Part print with two shaded views. Sizes in mm from the minimum x, y, z corner. A direction names the side the tool comes from. Round coordinates to 2 decimals unless told otherwise and drop trailing zeros. Loops run counter-clockwise (first coordinate to the right, second up) from the corner with the lowest first, then second, coordinate; pieces in that order, holes last. Notation, with made-up numbers: (20.25, 42) - (54.25, 42) arc R31 cw to (54.25, 70) - close; hole circle Ø4 at (57.5, 1.25). An arc over 180 degrees is marked (long way). Use a Markdown table: item, result.
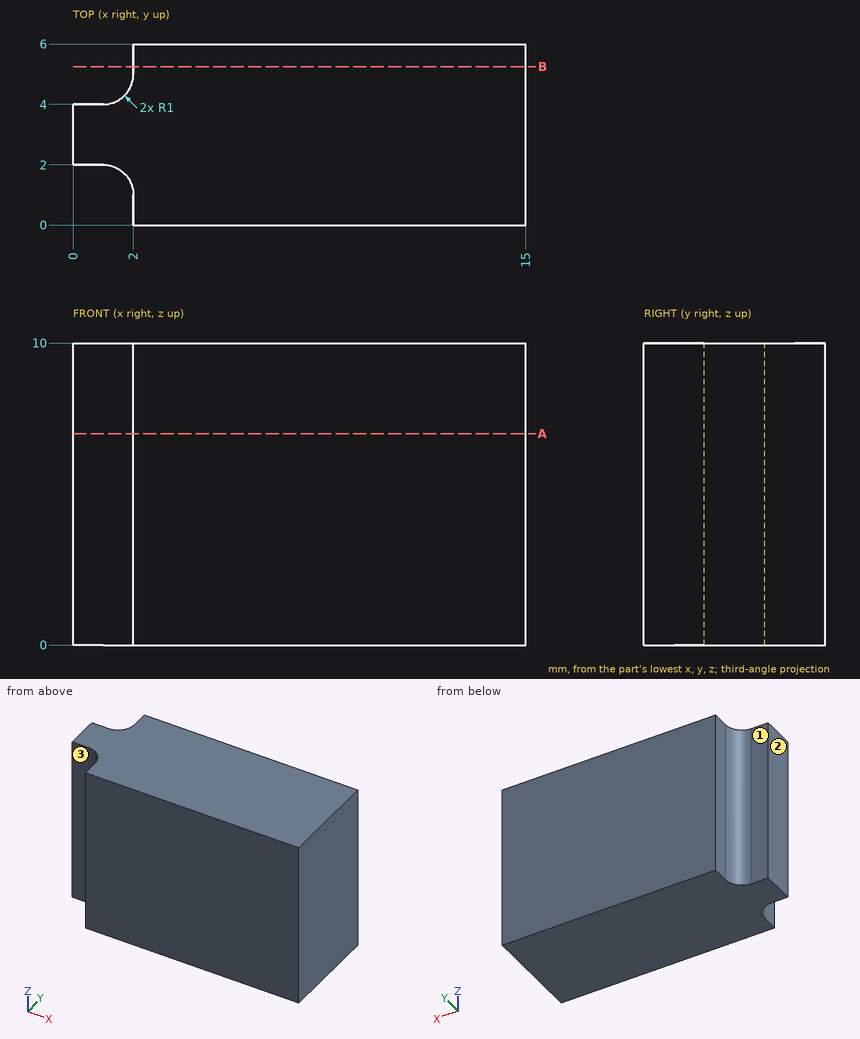
Q1. Drop flat-ended pins along their axis: pin 1 (0.5 mm diameter, centred on y = 5.5, z = 6, fed in from -X); pin 2 (6 mm diameter, centred on x = 10, z = 8, fed in from -Y); pin 3 (1.1 mm diameter, centred on x = 0.5, z = 5.5, fed in from +Y). Give the stop position or say it passes through.
Results found:
| item | result |
|---|---|
| pin 1 | stops at x = 2 |
| pin 2 | stops at y = 0 |
| pin 3 | stops at y = 4 |
Q2. Cut at B-B, the plane y = 5.25. List the corners of the cut face in (x, z).
Results found:
| item | result |
|---|---|
| outline | (2, 0) - (15, 0) - (15, 10) - (2, 10) - close |
Q3. Which spindle directions (+Z, -Z, +X, -X, +Y, -Y) get a long thin tool onto all of the face, cutting with end or side? Do the marked faces 1, 2 and 3. Say none if no direction does.
Results found:
| item | result |
|---|---|
| face 1 | +Z, -Z, -X, +Y |
| face 2 | +Z, -Z, -X, +Y, -Y |
| face 3 | +Z, -Z, -X, -Y |
Q4. Cut at A-A, the plane z = 7. List the corners of the cut face in (x, y).
Results found:
| item | result |
|---|---|
| outline | (0, 2) - (1, 2) arc R1 cw to (2, 1) - (2, 0) - (15, 0) - (15, 6) - (2, 6) - (2, 5) arc R1 cw to (1, 4) - (0, 4) - close |
Q5. Probe line 1 (X direction, y = 5.45, z = 3); line 2 (X direction, y = 4.15, z = 1.5); line 3 (Y direction, x = 1, z = 0.5). List the from-to ranges inside material, lowest first.
Results found:
| item | result |
|---|---|
| line 1 | x = 2 to 15 |
| line 2 | x = 1.53 to 15 |
| line 3 | y = 2 to 4 |
